Check sheet for the drawn part. Datum: minimum x, y, z corner. Units: mm. A direction names the side the tool comes from. Round coordinates to 2 decimals unless told otherwise and drop trailing zeros. Write each loop counter-clockwise with the first axis right and the second up, starting at its lowest first coordinate (ties: lowest second). Pieces come first, ordered by that corner, then holes. Notation, with made-up numbers: (79.25, -4) -> (108.25, -4) arc R23 cw to (108.25, 17) -> close; hole circle Ø7 at (43, 55.5). An arc over 180 degrees is marked (long way). Use a Markdown table: item, result.
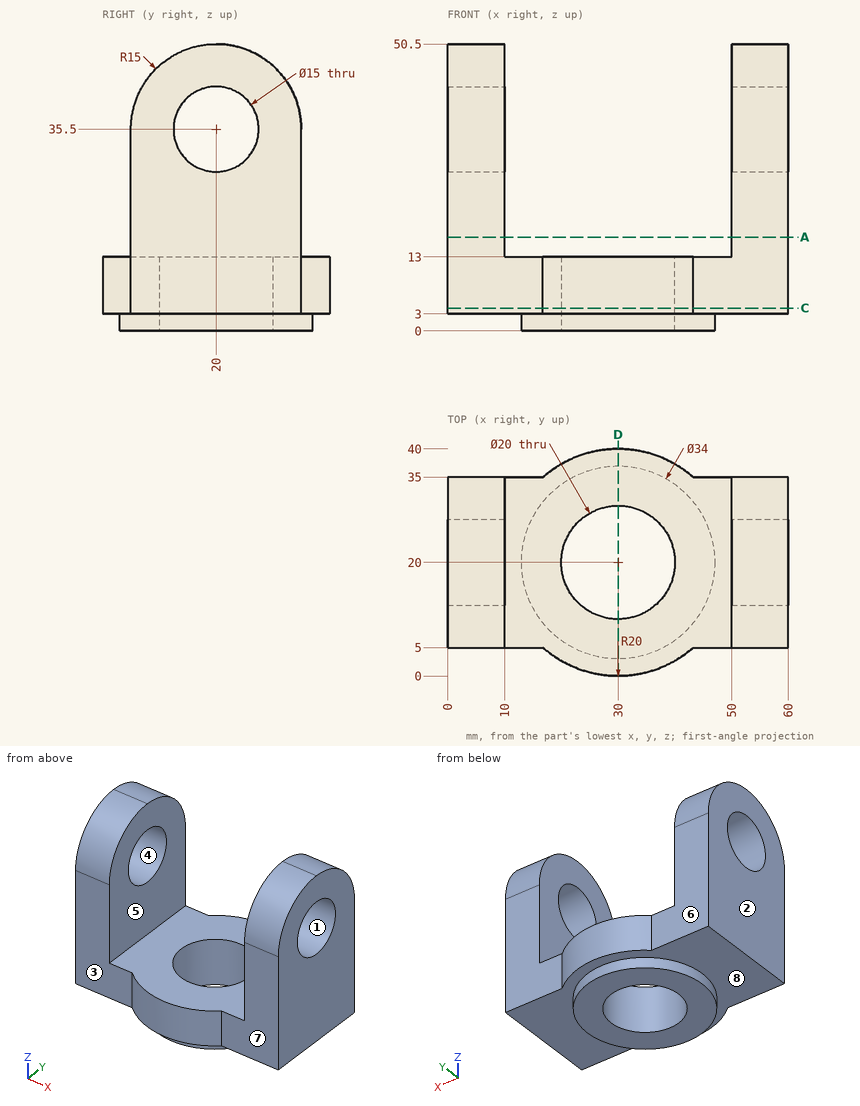
(1) Gauge pin test, flat ends, axial feed: pin 1 Ø13.5 at (y, z) = (20, 35.5) entering from -X; pin 2 Ø12 at (x, y) = (9, 13.5) entering from +Z; pin 3 Ø4 at (x, z) = (39, 11.5) entering from +Y (3 decimals); pin 4 Ø13.5 at (x, z) = (55.5, 15) entering from -Y. Record the tip position at first contact, or that the pin passes through.
A:
| item | result |
|---|---|
| pin 1 | passes through |
| pin 2 | stops at z = 50.49 |
| pin 3 | stops at y = 38.735 |
| pin 4 | stops at y = 5 |
(2) Section check C-C on z = 4. Record the cut outline in (x, y).
A:
| item | result |
|---|---|
| outline | (0, 5) -> (16.77, 5) arc R20 ccw to (43.23, 5) -> (60, 5) -> (60, 35) -> (43.23, 35) arc R20 ccw to (16.77, 35) -> (0, 35) -> close; hole circle Ø20 at (30, 20) |
(3) Access from +Z, -Z, +X, -X, +Y, -Y to the whole of each face (thin tool, end or side, straight path). Record for the marked faces 4, 5, 6, 7 and 8.
A:
| item | result |
|---|---|
| face 4 | +X, -X |
| face 5 | +Z, +Y, -Y |
| face 6 | +Z, -Z, -X, +Y |
| face 7 | +Z, -Z, +X, -Y |
| face 8 | -Z |
(4) Section check D-D on x = 30. Record the cut outline in (y, z), plus the area to 3 significant figures.
A:
| item | result |
|---|---|
| outline | (0, 3) -> (3, 3) -> (3, 0) -> (10, 0) -> (10, 13) -> (0, 13) -> close; (30, 0) -> (37, 0) -> (37, 3) -> (40, 3) -> (40, 13) -> (30, 13) -> close |
| area | 242 mm2 |
(5) Release check for a two-part mould opening along Y. For the marked faces 1, 2 and 3 record: +Y half, -Y half, draft (parallel to the pull), parting line (faces both ways), or undercut.
A:
| item | result |
|---|---|
| face 1 | undercut |
| face 2 | draft |
| face 3 | -Y half |
(6) Section check A-A on z = 16.5. Record the cut outline in (x, y), plus the area to 3 significant figures.
A:
| item | result |
|---|---|
| outline | (0, 5) -> (10, 5) -> (10, 35) -> (0, 35) -> close; (50, 5) -> (60, 5) -> (60, 35) -> (50, 35) -> close |
| area | 600 mm2 |
(7) Thickness scan on line 1 (Z direction, x = 52, y = 20); line 2 (X direction, y = 11, z = 22.5); line 3 (Y direction, x = 30, z = 4.5). Record the ranges inside material, lowest first.
A:
| item | result |
|---|---|
| line 1 | z = 3 to 28, 43 to 50.5 |
| line 2 | x = 0 to 10, 50 to 60 |
| line 3 | y = 0 to 10, 30 to 40 |
